Verification items for the finished model (mm, model axes). Face numbers are marked on the shaded views. A direction names the side the tool comes from. Round coordinates to 2 decimals unless told otherwise and drop trailing zeros. Order: outer loops, then holes, each group sorted by start corner. A loop starts at its lowest first (then second) coordinate and runs counter-clockwise, first axis right, second up. Notation, with made-up numbers: (-13.75, 83.25) -> (44.25, 83.25) arc R21 ccw to (44.25, 93.25) -> close; hole circle Ø2 at (66, 71). An arc over 180 degrees is marked (long way). Return JSON: item names as keys, results as strings. Group by question number.
Item 1: Scan lines: probe 1 along Z at (x, y) = (-15, -0.4); probe 2 along X at (y, z) = (0.7, 2.25); probe 3 along Y at (x, z) = (-27.5, -1.1). Record each from-to range of solid material in increasing order. Write a range as from..to.
Item 2: Access from +Z, -Z, +X, -X, +Y, -Y to the whole of each face (thin tool, end or side, straight path). Record for the marked faces 1, 2 and 3.
Item 3: Sectioned sample at C-C on x = -119. Record the cut outline in (y, z), plus the area to 3 significant figures.
Item 4: Sectioned sample at A-A on z = 0. Record the cut outline in (x, y).
Autodesk Inventor part; units mm, degrees
ref_plane "YZ Plane" through (0, 0, 0) normal (1, 0, 0) x (0, 1, 0)
ref_plane "XZ Plane" through (0, 0, 0) normal (0, 1, 0) x (-1, 0, 0)
ref_plane "XY Plane" through (0, 0, 0) normal (0, 0, 1) x (1, 0, 0)
sketch "Sketch1" plane through (0, 0, 0) normal (1, 0, 0) x (0, 1, 0)
  circle A0 centre (0, 0) radius 2.25
  dimension "d0" = 4.5
extrude "Extrusion1" add sketch "Sketch1" against normal blind 8
sketch "Sketch2" plane through (-8, 0, 0) normal (-1, 0, 0) x (0, 0, 1)
  circle A0 centre (0, 0) radius 2.75
  dimension "d6" = 5.5
extrude "Extrusion2" add sketch "Sketch2" along normal blind 129
sketch "Sketch3" plane through (-137, 0, 0) normal (-1, 0, 0) x (0, 0, 1)
  circle A0 centre (0, 0) radius 2.25
  dimension "d9" = 4.5
extrude "Extrusion3" add sketch "Sketch3" along normal blind 8
chamfer "Chamfer2" distance 0.25 angle 45 4 edges at (0, -2.25, 0) (-8, 0, -2.75) (-137, 0, -2.75) (-145, 0, -2.25)
properties part number "Ø5x145"
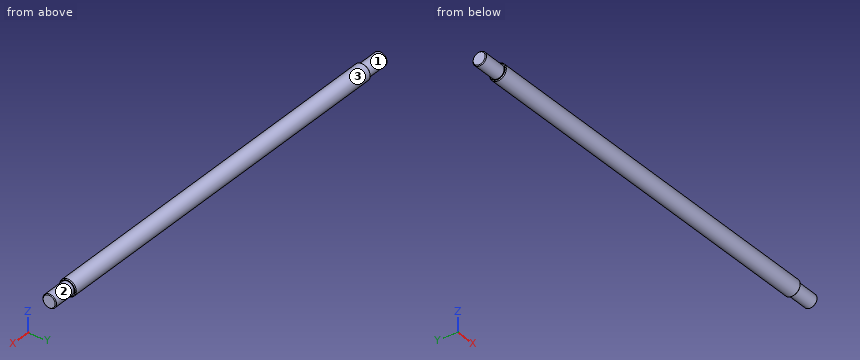
Recorded:
{
 "1": {"probe 1": "-2.72..2.72", "probe 2": "-137..-8", "probe 3": "-2.52..2.52"},
 "2": {"face 1": "-X", "face 2": "+X", "face 3": "+X, -X"},
 "3": {"outline": "circle Ø5.5 at (0, 0)", "area": "23.8 mm²"},
 "4": {"outline": "(-145, -2) -> (-144.75, -2.25) -> (-137, -2.25) -> (-137, -2.5) -> (-136.75, -2.75) -> (-8.25, -2.75) -> (-8, -2.5) -> (-8, -2.25) -> (-0.25, -2.25) -> (0, -2) -> (0, 2) -> (-0.25, 2.25) -> (-8, 2.25) -> (-8, 2.5) -> (-8.25, 2.75) -> (-136.75, 2.75) -> (-137, 2.5) -> (-137, 2.25) -> (-144.75, 2.25) -> (-145, 2) -> close"}
}
